Design review of the part built by this model. Coordinates are the model's own, in mm. A direction names the side the tool comes from. Round coordinates to 2 decimals unless told otherwise and drop trailing zeros. Loops run counter-clockwise (first coordinate to the right, second up) from the corner with the lowest first, then second, coordinate; pieces in that order, holes last. Notation, with made-up numbers: (14.5, -30.5) - (53.5, -30.5) arc R33 ccw to (53.5, 7.5) - close; hole circle Ø8 at (41, -36.5). An arc over 180 degrees is marked (long way). Return JSON: item names as keys, results as strings. Group by question number.
from build123d import *

# Parameters (mm, degrees)
F1_DEPTH = 12.7
F3_DEPTH = 762


# Not quite as in the source:
# - a feature names something its author has since deleted; it is built from what else it names


with BuildPart() as f1:
    # F0 (on Front) → F1 (new body)
    with BuildSketch(Plane.XZ):
        with BuildLine():
            Line((-457.2, 0), (0, 0))
            Line((0, 0), (762, 0))
            Line((762, 0), (762, 317.5))
            Line((762, 317.5), (0, 317.5))
            Line((0, 317.5), (0, 304.8))
            ThreePointArc((0, 304.8), (-37.1974387893, 214.9974387893), (-127, 177.8))
            Line((-127, 177.8), (-228.6, 177.8))
            ThreePointArc((-228.6, 177.8), (-318.4025612107, 214.9974387893), (-355.6, 304.8))
            Line((-355.6, 304.8), (-355.6, 457.2))
            Line((-355.6, 457.2), (-457.2, 457.2))
            Line((-457.2, 457.2), (-457.2, 0))
        make_face()
    extrude(amount=F1_DEPTH)

    # F2 (on face) → F3 (join, through all)
    with BuildSketch(Plane.YZ.offset(762)):
        Polygon((-12.7, 317.5), (0, 317.5), (-12.7, 322.7605122421), align=None)
    extrude(amount=-F3_DEPTH)


solid = f1.part
Q1. Tool access review of faces 1 (the cylindrical face through (-36.215, -6.261, 215.99)), 2 (the flat face through (161, -12.7, 181)): name each direction out of +Z, -Z, +X, -X, +Y, -Y from which nothing blocks a thin tool from reaching the whole face with its end or side.
Q2. Draft analysis for pull direction X (two halves, no side actions). For faces 3 (the cylindrical face through (-317.41, -6.261, 214.015)), 4 (the flat face through (144, 0, 181)), state which applies: pulls with the +X half, pulls with the -X half, needs draft (parallel to the pull), parting line crosses it, or undercut.
Q3. Add section A-A, the plane z = 246. State the section outline as (x, y) points, plus the area to 3 significant figures.
Q4. For line 1 (X direction, y = -10.5, z = 230); line 2 (X direction, y = -6.25, z = 405); line 3 (X direction, y = -5.75, z = 193.5), list the stretches that pass through material, from the lowest coordinate up.
Q5. Add section D-D, the plane z = 196.5. State the section outline as (x, y) points, plus the area to 3 significant figures.
Q6. Add section B-B, the plane y = -7. State the section outline as (x, z) points, plus the area to 3 significant figures.
Q7. Insertion check: pin 1 Ø4 at (x, y) = (102, -7.5) entering from -Z; pin 2 Ø2 at (y, z) = (-4, 321) entering from +X. Each pin has a flat end and moves straight along its axis. Give the tip position at first contact, or say it passes through.
Q8. Add section C-C, the plane x = 25.5. State the section outline as (y, z) points.
Evaluation:
{
 "1": {"face 1": "+Z, +Y, -Y", "face 2": "+Z, -Z, +X, -X, -Y"},
 "2": {"face 3": "undercut", "face 4": "needs draft"},
 "3": {"outline": "(-457.2, -12.7) - (-341.17, -12.7) - (-341.17, 0) - (-457.2, 0) - close; (-14.43, -12.7) - (762, -12.7) - (762, 0) - (-14.43, 0) - close", "area": "11,300 mm²"},
 "4": {"line 1": "-457.2 to -331.24, -24.36 to 762", "line 2": "-457.2 to -355.6", "line 3": "-457.2 to -289.77, -65.83 to 762"},
 "5": {"outline": "(-457.2, -12.7) - (-294.93, -12.7) - (-294.93, 0) - (-457.2, 0) - close; (-60.67, -12.7) - (762, -12.7) - (762, 0) - (-60.67, 0) - close", "area": "12,500 mm²"},
 "6": {"outline": "(-457.2, 0) - (762, 0) - (762, 320.4) - (0, 320.4) - (0, 304.8) arc R127 cw to (-127, 177.8) - (-228.6, 177.8) arc R127 cw to (-355.6, 304.8) - (-355.6, 457.2) - (-457.2, 457.2) - close", "area": "361,000 mm²"},
 "7": {"pin 1": "z = 0", "pin 2": "x = -355.6"},
 "8": {"outline": "(-12.7, 0) - (0, 0) - (0, 317.5) - (-12.7, 322.76) - close"}
}
